Part model, mm, in its own coordinate system. A direction names the side the tool comes from. Coordinates: 2 decimals unless noted, no trailing zeros. Order: outer loops, then holes, each group sorted by start corner. A loop starts at its lowest first (then second) coordinate and runs counter-clockwise, first axis right, second up. Notation, with made-up numbers: (76.25, 21) - (99.25, 21) arc R25 ccw to (99.25, 46) - close; hole circle Ø2 at (25.5, 16). An arc over 180 degrees is marked (long way). Use a Markdown table: item, result. Add a question column.
1) Drop flat-ended pins along their axis: P1, Ø1.5, axis at y = 86.5, z = 1.5, coming from the -X side; P2, Ø1.8, axis at y = 78.5, z = 2, coming from the -X side; P3, Ø1, axis at x = -20.5, z = 1.5, coming from the -Y side. Give the stop position or say it passes through.
2) Tool access for faces 1 (the face through (-17, 32.016, 2)), 2 (the face through (-16.03, 133.96, 1.58)): list every direction of +Z, -Z, +X, -X, +Y, -Y with a clear straight run to the whole face (end or side of a thin tool).
3) Wall check: L1, parallel to X at y = 61.5, z = 3.2; L2, parallel to Y at x = -29.5, z = 3.25; L3, parallel to X at y = 102.5, z = 1.1. Give the ranges that are in metal, low to high. Write a range as [from, to].
4) Saw through at A-A on x = -30. List the corners of the cut face in (y, z), then the cut area to 3 significant figures.
5) Saw through at C-C on z = 1. List the corners of the cut face in (x, y).
6) Saw through at B-B on y = 111.5. List the corners of the cut face in (x, z), then the cut area to 3 significant figures.
7) Two-plate mould, pull along X, no slides. Class faces 3 (the face through (-17, 130.016, 2)), 4 (the face through (13, 82, 3.5)), 5 (the face through (-41.45, 82, 2)), 6 (the face through (-45.4, 80.23, 1.58)): +X half, -X half, draft (parallel to the pull), parting line (faces both ways), or undercut.
```python
from build123d import *

# Parameters (mm, degrees)
BOSS_EXTRUDE1_DEPTH = 3.5
CHAMFER1_SIZE       = 7
CHAMFER1_SIZE2      = 3.116600797


with BuildPart() as part:
    # Sketch1 → Boss-Extrude1 (new body)
    with BuildSketch(Plane.XY):
        Polygon((7.962573201, 32.016439516), (15.870478339, 24.620213101), (-48.846502793, 24.620213101), (-41.450276378, 32.016439516), align=None)
        Polygon((-48.846502793, 137.412665932), (-41.450276378, 130.016439516), (-41.450276378, 32.016439516), (-48.846502793, 24.620213101), align=None)
        Polygon((15.870478339, 137.412665932), (-48.846502793, 137.412665932), (-41.450276378, 130.016439516), (7.962573201, 130.016439516), align=None)
        Polygon((15.870478339, 137.412665932), (15.870478339, 24.620213101), (7.962573201, 32.016439516), (7.962573201, 130.016439516), align=None)
    extrude(amount=BOSS_EXTRUDE1_DEPTH)

    # Chamfer1
    chamfer1_edges = [part.edges().sort_by_distance(p)[0] for p in [
        (-48.846502793, 81.016439516, 0),
        (-16.488012227, 137.412665932, 0),
        (15.870478339, 81.016439516, 0),
        (-16.488012227, 24.620213101, 0),
    ]]
    chamfer1_side = [part.faces().sort_by_distance(p)[0] for p in [
        (-16.488012227, 25.920614003, 0),
    ]]
    chamfer(chamfer1_edges, length=CHAMFER1_SIZE, length2=CHAMFER1_SIZE2, reference=chamfer1_side[0])


solid = part.part
```
Results are:
| question | item | result |
|---|---|---|
| 1 | P1 | x = -46.9 |
| 1 | P2 | x = -48.36 |
| 1 | P3 | y = 27.13 |
| 2 | face 1 | +Z, -Z |
| 2 | face 2 | -Z, +X, -X, +Y |
| 3 | L1 | [-48.85, -41.45], [7.96, 15.87] |
| 3 | L2 | [24.62, 32.02], [130.02, 137.41] |
| 3 | L3 | [-44.32, -41.45], [7.96, 11.34] |
| 4 | outline | (24.62, 3.12) - (31.62, 0) - (32.02, 0) - (32.02, 3.5) - (24.62, 3.5) - close; (130.02, 0) - (130.41, 0) - (137.41, 3.12) - (137.41, 3.5) - (130.02, 3.5) - close |
| 4 | area | 30.0 mm2 |
| 5 | outline | (-44.09, 29.37) - (11.12, 29.37) - (11.12, 132.66) - (-44.09, 132.66) - close; hole (-41.45, 32.02) - (7.96, 32.02) - (7.96, 130.02) - (-41.45, 130.02) - close |
| 6 | outline | (-48.85, 3.12) - (-41.85, 0) - (-41.45, 0) - (-41.45, 3.5) - (-48.85, 3.5) - close; (7.96, 0) - (8.87, 0) - (15.87, 3.12) - (15.87, 3.5) - (7.96, 3.5) - close |
| 6 | area | 31.7 mm2 |
| 7 | face 3 | undercut |
| 7 | face 4 | draft |
| 7 | face 5 | undercut |
| 7 | face 6 | -X half |
